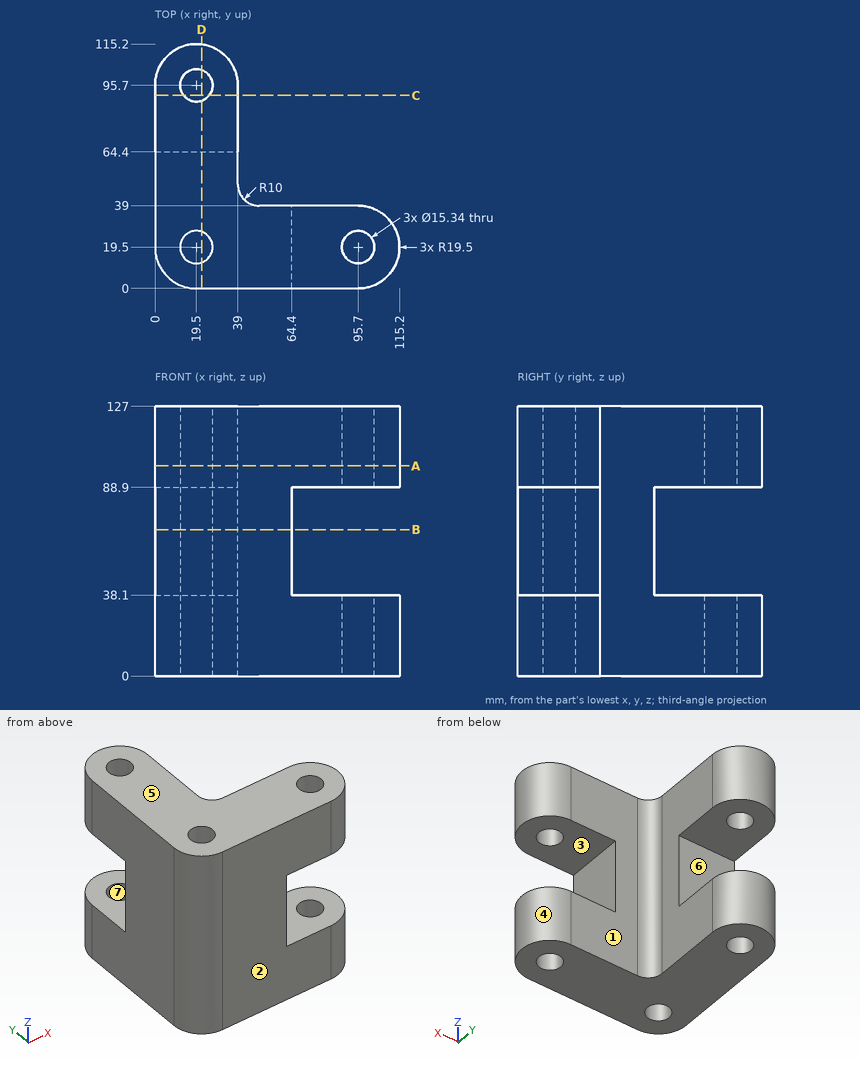
For this review, use the dimensioned drawing (mm, ordinates from the lowest corner) and the shaded views. A direction names the side the tool comes from. Coordinates: 2 decimals unless noted, no trailing zeros. Write each loop counter-clockwise with the first axis right and the second up, starting at its lowest first coordinate (ties: lowest second). Pieces come first, ordered by that corner, then holes. Notation, with made-up numbers: (-4, 32.25) -> (55, 32.25) arc R32 ccw to (55, 65.25) -> close; hole circle Ø5 at (24.25, -10.5). An arc over 180 degrees is marked (long way). Write each question's results on one line, items separated by ' | '. Start each with the question number.
(1) Take a section at A-A on z = 99. Write out the cut boundary in (x, y), and give its area (3 significant figures).
(2) The part is to be moulded in two halves that separate along Y. For the marked faces 4, 5, 6 and 7, say which applies: pulls with the +Y half, pulls with the -Y half, needs draft (parallel to the pull), parting line crosses it, or undercut.
(3) Clearance check with flat-ended pins moving along their axes: P1, Ø10, axis at y = 31.5, z = 45.5, coming from the +X side; P2, Ø12, axis at x = 41, z = 36, coming from the +Y side; P3, Ø8, axis at x = 78.5, z = 40, coming from the +Y side. State where each tip first meets the part, or that it passes through.
(4) Take a section at D-D on x = 22. Write out the cut boundary in (y, z), and give its area (3 significant figures).
(5) For line 1 along Y through (x, z) = (19.5, 104.5); line 2 along Z through (x, y) = (29.5, 101); line 3 along X through (y, z) = (14, 14), list the stretches that pass through material, from the lowest coordinate up. Write a range as from..to.
(6) Take a section at C-C on y = 91. Write out the cut boundary in (x, z).
(7) Tool access review of the marked faces 1, 2 and 3: name each direction out of +Z, -Z, +X, -X, +Y, -Y from which nothing blocks a thin tool from reaching the whole face with its end or side.
(8) Take a section at B-B on z = 69. Write out the cut boundary in (x, y).
Results found:
1) outline: (0, 19.5) arc R19.5 ccw to (19.5, 0) -> (95.7, 0) arc R19.5 ccw to (95.7, 39) -> (49, 39) arc R10 cw to (39, 49) -> (39, 95.7) arc R19.5 ccw to (0, 95.7) -> close; hole circle Ø15.34 at (19.5, 19.5); hole circle Ø15.34 at (19.5, 95.7); hole circle Ø15.34 at (95.7, 19.5) | area: 6,520 mm2
2) face 4: parting line crosses it | face 5: needs draft | face 6: pulls with the +Y half | face 7: undercut
3) P1: stops at x = 64.4 | P2: stops at y = 107.53 | P3: stops at y = 39
4) outline: (0, 0) -> (12.25, 0) -> (12.25, 127) -> (0, 127) -> close; (26.75, 0) -> (88.45, 0) -> (88.45, 38.1) -> (64.4, 38.1) -> (64.4, 88.9) -> (88.45, 88.9) -> (88.45, 127) -> (26.75, 127) -> close; (102.95, 0) -> (115.04, 0) -> (115.04, 38.1) -> (102.95, 38.1) -> close; (102.95, 88.9) -> (115.04, 88.9) -> (115.04, 127) -> (102.95, 127) -> close | area: 9,090 mm2
5) line 1: y = 0..11.83, 27.17..88.03, 103.37..115.2 | line 2: z = 0..38.1, 88.9..127 | line 3: x = 0.79..14.15, 24.85..90.35, 101.05..114.41
6) outline: (0, 0) -> (13.44, 0) -> (13.44, 38.1) -> (0, 38.1) -> close; (0, 88.9) -> (13.44, 88.9) -> (13.44, 127) -> (0, 127) -> close; (25.56, 0) -> (39, 0) -> (39, 38.1) -> (25.56, 38.1) -> close; (25.56, 88.9) -> (39, 88.9) -> (39, 127) -> (25.56, 127) -> close
7) face 1: +Z, -Z, +X, +Y | face 2: +Z, -Z, +X, -X, -Y | face 3: +X, +Y, -Y
8) outline: (0, 19.5) arc R19.5 ccw to (19.5, 0) -> (64.4, 0) -> (64.4, 39) -> (49, 39) arc R10 cw to (39, 49) -> (39, 64.4) -> (0, 64.4) -> close; hole circle Ø15.34 at (19.5, 19.5)
